```python
from build123d import *

# Parameters (mm, degrees)
SKETCH_W      = 8
SKETCH_H      = 10
PAD_DEPTH     = 0.8
SKETCH001_W   = 2.75
SKETCH001_H   = 2.333333
SKETCH001_H_2 = 2.333334
POCKET_DEPTH  = 5


with BuildPart() as part:
    # Sketch → Pad (new body)
    with BuildSketch(Plane.XZ):
        Rectangle(SKETCH_W, SKETCH_H)
    extrude(amount=PAD_DEPTH)

    # Sketch001 (on Face6 of Pad) → Pocket (cut)
    with BuildSketch(Plane.XZ.offset(0.8)):
        with Locations((-1.625, 2.833334)):
            Rectangle(SKETCH001_W, SKETCH001_H)
        with Locations((-1.625, 0)):
            Rectangle(SKETCH001_W, SKETCH001_H_2)
        with Locations((-1.625, -2.833334)):
            Rectangle(SKETCH001_W, SKETCH001_H)
        with Locations((1.625, 2.833334)):
            Rectangle(SKETCH001_W, SKETCH001_H)
        with Locations((1.625, 0)):
            Rectangle(SKETCH001_W, SKETCH001_H_2)
        with Locations((1.625, -2.833334)):
            Rectangle(SKETCH001_W, SKETCH001_H)
    extrude(amount=-POCKET_DEPTH, mode=Mode.SUBTRACT)


solid = part.part
```
Verification items for the finished model (mm, model axes). Round coordinates to 2 decimals unless told otherwise and drop trailing zeros. Order: outer loops, then holes, each group sorted by start corner. A loop starts at its lowest first (then second) coordinate and runs counter-clockwise, first axis right, second up. Notation, with made-up numbers: (39, 88.25) -> (46, 88.25) arc R18 cw to (46, 98.25) -> close; hole circle Ø3 at (-37.75, -37.5). An arc over 180 degrees is marked (long way). Put each result on its own line as item: value. Start each with the question number.
(1) Material ranges on line 1 along Z through (x, y) = (-0.5, -0.3); line 2 along X through (y, z) = (-0.45, -0.25), recorded low to high.
(2) Section check C-C (y = -0.65). Enter the section's corners in (x, z), then the cut area to 3 significant figures.
(3) Section check B-B (z = -3.25). Enter the section's corners in (x, y).
(4) Section check A-A (x = 1.75). Enter the section's corners in (y, z).
Completed:
1. line 1: z = -5 to -4, -1.67 to -1.17, 1.17 to 1.67, 4 to 5
1. line 2: x = -4 to -3, -0.25 to 0.25, 3 to 4
2. outline: (-4, -5) -> (4, -5) -> (4, 5) -> (-4, 5) -> close; hole (-3, -4) -> (-0.25, -4) -> (-0.25, -1.67) -> (-3, -1.67) -> close; hole (-3, -1.17) -> (-0.25, -1.17) -> (-0.25, 1.17) -> (-3, 1.17) -> close; hole (-3, 1.67) -> (-0.25, 1.67) -> (-0.25, 4) -> (-3, 4) -> close; hole (0.25, -4) -> (3, -4) -> (3, -1.67) -> (0.25, -1.67) -> close; hole (0.25, -1.17) -> (3, -1.17) -> (3, 1.17) -> (0.25, 1.17) -> close; hole (0.25, 1.67) -> (3, 1.67) -> (3, 4) -> (0.25, 4) -> close
2. area: 41.5 mm2
3. outline: (-4, -0.8) -> (-3, -0.8) -> (-3, 0) -> (-4, 0) -> close; (-0.25, -0.8) -> (0.25, -0.8) -> (0.25, 0) -> (-0.25, 0) -> close; (3, -0.8) -> (4, -0.8) -> (4, 0) -> (3, 0) -> close
4. outline: (-0.8, -5) -> (0, -5) -> (0, -4) -> (-0.8, -4) -> close; (-0.8, -1.67) -> (0, -1.67) -> (0, -1.17) -> (-0.8, -1.17) -> close; (-0.8, 1.17) -> (0, 1.17) -> (0, 1.67) -> (-0.8, 1.67) -> close; (-0.8, 4) -> (0, 4) -> (0, 5) -> (-0.8, 5) -> close
